Design review of the part built by this model. Coordinates are the model's own, in mm. Give positions to 0.01 mm unless a question says otherwise; leave off trailing zeros. Write each loop counter-clockwise with the first axis right and the second up, starting at its lowest first coordinate (ties: lowest second). Pieces come first, ordered by that corner, then holes. Notation, with made-up numbers: M -33,22 L 21,22 A22 ccw 21,55 Z; hole C 14,3 d7. An arc over 180 degrees is marked long. Answer in a Markdown table with one row per item.
```python
from build123d import *

# Parameters (mm, degrees)
SKETCH1_R           = 5
SKETCH1_R_2         = 4
BOSS_EXTRUDE1_DEPTH = 2.9


with BuildPart() as part:
    # Sketch1 → Boss-Extrude1 (new body)
    with BuildSketch(Plane(origin=(116, 0, 0), x_dir=(0, 0, -1), z_dir=(1, 0, 0))):
        Polygon((-135, 2.9), (-115, 2.9), (-115, 0.5), (-114.5, 0), (-85.5, 0), (-85, 0.5), (-85, 2.9), (-15, 2.9), (-15, 0.5), (-14.5, 0), (14.5, 0), (15, 0.5), (15, 2.9), (70, 2.9), (70, 0.5), (70.5, 0), (99.5, 0), (100, 0.5), (100, 2.9), (135, 2.9), (135, 18.725), (137.9, 18.725), (137.9, 34.475), (135, 34.475), (135, 50.325), (137.9, 50.325), (137.9, 66.075), (135, 66.075), (135, 81.9), (100, 81.9), (100, 84.3), (99.5, 84.8), (70.5, 84.8), (70, 84.3), (70, 81.9), (-85, 81.9), (-85, 84.3), (-85.5, 84.8), (-114.5, 84.8), (-115, 84.3), (-115, 81.9), (-135, 81.9), (-135, 66.075), (-137.9, 66.075), (-137.9, 50.325), (-135, 50.325), (-135, 34.475), (-137.9, 34.475), (-137.9, 18.725), (-135, 18.725), align=None)
        with Locations((-113, 45)):
            Circle(SKETCH1_R, mode=Mode.SUBTRACT)
        with Locations((-93, 45)):
            Circle(SKETCH1_R, mode=Mode.SUBTRACT)
        with Locations((-73, 45)):
            Circle(SKETCH1_R_2, mode=Mode.SUBTRACT)
        with Locations((-53, 45)):
            Circle(SKETCH1_R_2, mode=Mode.SUBTRACT)
    extrude(amount=BOSS_EXTRUDE1_DEPTH)


solid = part.part
```
1) Add section C-C (x = 117.2). Count the separate pieces of the cut face and the enclosed holes in it, and give its area (3 significant figures).
Geometry says:
| item | result |
|---|---|
| separate pieces | 1 |
| enclosed holes | 4 |
| area | 21,700 mm^2 |
2) To check wall thickness, follow probe 1 along Z at (x, y) = (117.25, 45.5); probe 2 along Y at (x, z) = (118.25, 93); probe 3 along Z at (x, y) = (116.45, 47.5). State the ranges of each line that lie inside material, in increasing order. Write a range as [from, to].
Geometry says:
| item | result |
|---|---|
| probe 1 | [-135, 49.03], [56.97, 69.03], [76.97, 88.03], [97.97, 108.03], [117.97, 135] |
| probe 2 | [0, 40], [50, 84.8] |
| probe 3 | [-135, 49.88], [56.12, 69.88], [76.12, 88.67], [97.33, 108.67], [117.33, 135] |
3) Add section A-A (z = 73). Write out the cut boundary in (x, y), and give its area (3 significant figures).
Geometry says:
| item | result |
|---|---|
| outline | M 116,2.9 L 118.9,2.9 L 118.9,41 L 116,41 Z; M 116,49 L 118.9,49 L 118.9,81.9 L 116,81.9 Z |
| area | 206 mm^2 |
4) The part is to be moulded in two halves that separate along Y. For faces 1 (the face through (117.43, 43.468, 69.305)), 2 (the face through (116, 43, 2)), say which applies: released by +Y, released by -Y, zero draft, split by the parting line, or undercut.
Geometry says:
| item | result |
|---|---|
| face 1 | undercut |
| face 2 | zero draft |
5) Insertion check: P1, Ø1.5, axis at x = 118, z = 137, coming from the -Y side (3 decimals); P2, Ø1.2, axis at x = 117.5, y = 83, coming from the -Z side; P3, Ø0.9, axis at x = 117.5, z = -109.5, coming from the +Y side. Each pin has a flat end and moves straight along its axis. Give the tip position at first contact, or say it passes through.
Geometry says:
| item | result |
|---|---|
| P1 | y = 18.725 |
| P2 | z = -100 |
| P3 | y = 81.9 |
6) Add section B-B (y = 45). Write out the cut boundary in (x, z), and give its area (3 significant figures).
Geometry says:
| item | result |
|---|---|
| outline | M 116,-135 L 118.9,-135 L 118.9,49 L 116,49 Z; M 116,57 L 118.9,57 L 118.9,69 L 116,69 Z; M 116,77 L 118.9,77 L 118.9,88 L 116,88 Z; M 116,98 L 118.9,98 L 118.9,108 L 116,108 Z; M 116,118 L 118.9,118 L 118.9,135 L 116,135 Z |
| area | 679 mm^2 |
7) Add section D-D (z = 112). Write out the cut boundary in (x, y).
Geometry says:
| item | result |
|---|---|
| outline | M 116,0 L 118.9,0 L 118.9,40.1 L 116,40.1 Z; M 116,49.9 L 118.9,49.9 L 118.9,84.8 L 116,84.8 Z |
